Autodesk Fusion 360 part; units mm, degrees
sketch "Sketch1" plane through (0, 0, 0) normal (0, 0, 1) x (1, 0, 0)
  line L0 (-47.5, 47.5) -> (47.5, 47.5)
  line L1 (47.5, 47.5) -> (47.5, -47.5)
  line L2 (47.5, -47.5) -> (-47.5, -47.5)
  line L3 (-47.5, -47.5) -> (-47.5, 47.5)
  line L4 (-47.5, 47.5) -> (47.5, -47.5) construction
  line L5 (-47.5, -47.5) -> (47.5, 47.5) construction
  circle A0 centre (0, 0) radius 35.2
  dimension "d1" = 95
  dimension "d2" = 95
  dimension "d3" = 70.4
extrude "Extrude1" add sketch "Sketch1" along normal blind 10
sketch "Sketch2" plane through (0, 0, 10) normal (0, 0, 1) x (-1, 0, 0)
  circle A0 centre (0, 0) radius 35.2
  line L0 (47.5, 47.5) -> (-47.5, 47.5)
  line L1 (-47.5, 47.5) -> (-47.5, -47.5)
  line L2 (-47.5, -47.5) -> (47.5, -47.5)
  line L3 (47.5, -47.5) -> (47.5, 47.5)
  line L4 (42.5, 0) -> (-42.5, 0) construction
  line L5 (0, -42.5) -> (0, 42.5) construction
  point P0 (0, -42.5)
  point P1 (42.5, 0)
  point P2 (0, 42.5)
  point P3 (-42.5, 0)
  dimension "d7" = 5
  dimension "d8" = 5
  dimension "d9" = 5
  dimension "d10" = 5
hole "Hole1" at (-42.5, 0, 10) at (0, 42.5, 10) at (42.5, 0, 10) at (0, -42.5, 10) direction (0, 0, -1) diameter 4.5 depth 15 tip angle 118 counterbore diameter 8 counterbore depth 4
sketch "Sketch3" plane through (0, 0, 10) normal (0, 0, 1) x (-1, 0, 0)
  circle A0 centre (-42.5, 0) radius 4
  circle A1 centre (42.5, 0) radius 4
  circle A2 centre (0, -42.5) radius 4
  circle A3 centre (0, 42.5) radius 4
  circle A4 centre (0, 0) radius 35.2
  line L0 (47.5, 47.5) -> (-47.5, 47.5)
  line L1 (-47.5, 47.5) -> (-47.5, -47.5)
  line L2 (-47.5, -47.5) -> (47.5, -47.5)
  line L3 (47.5, -47.5) -> (47.5, 47.5)
  line L4 (37.5, -37.5) -> (37.5, 37.5) construction
  line L5 (37.5, 37.5) -> (-37.5, 37.5) construction
  line L6 (-37.5, 37.5) -> (-37.5, -37.5) construction
  line L7 (-37.5, -37.5) -> (37.5, -37.5) construction
  point P0 (37.5, -37.5)
  point P1 (-37.5, -37.5)
  point P2 (-37.5, 37.5)
  point P3 (37.5, 37.5)
  dimension "d16" = 10
  dimension "d17" = 10
  dimension "d18" = 10
  dimension "d19" = 10
hole "Hole2" at (-37.5, 37.5, 10) at (37.5, 37.5, 10) at (37.5, -37.5, 10) at (-37.5, -37.5, 10) direction (0, 0, -1) diameter 11 end through all
equation "d2 = d1"
equation "d8 = d7"
equation "d9 = d7"
equation "d10 = d7"
equation "d17 = d16"
equation "d18 = d16"
equation "d19 = d16"
Input: part model. Units: mm. Frame: model coordinates. A direction names the side the tool comes from. Round coordinates to 2 decimals unless told otherwise and drop trailing zeros. Loops run counter-clockwise (first coordinate to the right, second up) from the corner with the lowest first, then second, coordinate; pieces in that order, holes last. Notation, with made-up numbers: (72.25, 31) -> (116.25, 31) arc R26 cw to (116.25, 59) -> close; hole circle Ø7 at (86, 31). An arc over 180 degrees is marked (long way). Use one line per item in the form item = value. Start each with the question number.
Item 1: Section query B-B on x = 0. Return the cut outline in (y, z), then the cut area to 3 significant figures.
Item 2: Set-up query: faces 4 (the face through (-41, -2, 6)), 5 (the face through (40.27, 0.29, 2.96)). Return all of +Z, -Z, +X, -X, +Y, -Y with unobstructed straight access to the full face (end or side cutting, diameter ignored); none if empty.
Item 3: Section query C-C on y = -5.5. Return the cut outline in (x, z), then the cut area to 3 significant figures.
Item 4: Section query A-A on z = 8.25. Count the separate pieces of the cut face and the enclosed holes in it, then the cut area to 3 significant figures.
Item 5: Mould query, pull axis Y, two halves, no side actions, for faces 1 (the face through (32.047, -36.784, 4.93)), 2 (the face through (1, -47.5, 5)), 3 (the face through (-47.5, -1, 5)). Classes: pulls with the +Y half, pulls with the -Y half, needs draft (parallel to the pull), parting line crosses it, or undercut.
Item 6: Material intervals for L1, parallel to Y at x = 37, z = 5.5; L2, parallel to X at y = 37.5, z = 6; L3, parallel to Y at x = 0, z = 1.8, sorted ascending. Write a range as from..to.
Item 7: Contact query for a flat-ended pin moving along its axis: pin 1 Ø6.5 at (x, y) = (43, -0.5) entering from +Z. Output: stop coordinate, or through.
Ans:
q1.outline = (-47.5, 0) -> (-44.75, 0) -> (-44.75, 6) -> (-46.5, 6) -> (-46.5, 10) -> (-47.5, 10) -> close; (-40.25, 0) -> (-35.2, 0) -> (-35.2, 10) -> (-38.5, 10) -> (-38.5, 6) -> (-40.25, 6) -> close; (35.2, 0) -> (40.25, 0) -> (40.25, 6) -> (38.5, 6) -> (38.5, 10) -> (35.2, 10) -> close; (44.75, 0) -> (47.5, 0) -> (47.5, 10) -> (46.5, 10) -> (46.5, 6) -> (44.75, 6) -> close
q1.area = 128 mm^2
q2.face_4 = +Z
q2.face_5 = +Z, -Z
q3.outline = (-47.5, 0) -> (-34.77, 0) -> (-34.77, 10) -> (-47.5, 10) -> close; (34.77, 0) -> (47.5, 0) -> (47.5, 10) -> (34.77, 10) -> close
q3.area = 255 mm^2
q4.separate_pieces = 1
q4.enclosed_holes = 9
q4.area = 4,550 mm^2
q5.face_1 = undercut
q5.face_2 = pulls with the -Y half
q5.face_3 = needs draft
q6.L1 = -47.5..-42.98, -32.02..32.02, 42.98..47.5
q6.L2 = -47.5..-43, -32..32, 43..47.5
q6.L3 = -47.5..-44.75, -40.25..-35.2, 35.2..40.25, 44.75..47.5
q7.pin_1 = 6
